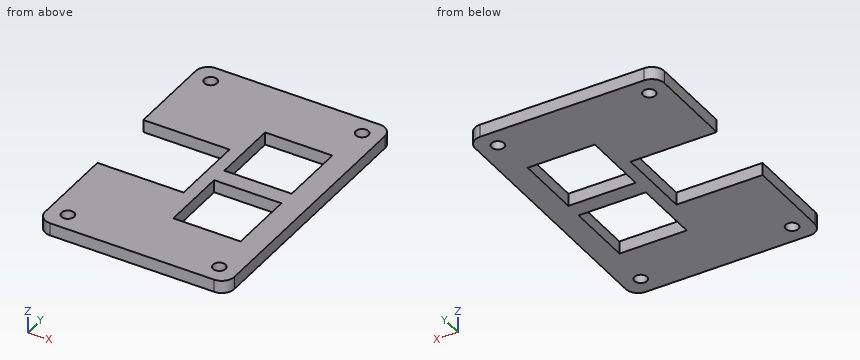
Autodesk Inventor part; units mm, degrees
ref_plane "YZ Plane" through (0, 0, 0) normal (1, 0, 0) x (0, 1, 0)
ref_plane "XZ Plane" through (0, 0, 0) normal (0, 1, 0) x (-1, 0, 0)
ref_plane "XY Plane" through (0, 0, 0) normal (0, 0, 1) x (1, 0, 0)
sketch "Эскиз1" plane through (0, 0, 0) normal (0, 0, 1) x (1, 0, 0)
  arc A0 (22.5, 29.5) -> (19.5, 32.5) centre (19.5, 29.5) ccw
  line L0 (22.5, -29.5) -> (22.5, 29.5)
  arc A1 (19.5, -32.5) -> (22.5, -29.5) centre (19.5, -29.5) ccw
  line L1 (-19.5, -32.5) -> (19.5, -32.5)
  line L2 (19.5, 32.5) -> (-19.5, 32.5)
  arc A2 (-19.5, 32.5) -> (-22.5, 29.5) centre (-19.5, 29.5) ccw
  line L3 (-22.5, 29.5) -> (-22.5, 9)
  line L4 (-22.5, -9) -> (-22.5, -29.5)
  arc A3 (-22.5, -29.5) -> (-19.5, -32.5) centre (-19.5, -29.5) ccw
  circle A4 centre (-18, -28) radius 1.5
  circle A5 centre (18, -28) radius 1.5
  circle A6 centre (18, 28) radius 1.5
  circle A7 centre (-18, 28) radius 1.5
  line L5 (-2, 9) -> (-20, 9)
  line L6 (-22.5, 9) -> (-20, 9)
  line L7 (-2, -9) -> (-2, 9)
  line L8 (-20, -9) -> (-2, -9)
  line L9 (-20, -9) -> (-22.5, -9)
  line L10 (1, -2) -> (1, -18)
  line L11 (1, -18) -> (17, -18)
  line L12 (17, -18) -> (17, -2)
  line L13 (17, -2) -> (1, -2)
  line L14 (1, 18) -> (1, 2)
  line L15 (1, 2) -> (17, 2)
  line L16 (17, 2) -> (17, 18)
  line L17 (17, 18) -> (1, 18)
  point P0 (0, 0)
extrude "Выдавливание1" add sketch "Эскиз1" along normal blind 3
properties part number "level2_up"
Can you work these out from the model? Positions are in its coordinate system, mm. Give positions to 0.01 mm unless a question says otherwise; leave off trailing zeros. Write each loop counter-clockwise with the first axis right and the second up, starting at its lowest first coordinate (ties: lowest second). Pieces come first, ordered by that corner, then holes. Notation, with made-up numbers: (-9.75, -31.75) -> (15.25, -31.75) arc R27 cw to (15.25, -3.75) -> close; hole circle Ø8 at (-27.75, -19). An arc over 180 degrees is marked (long way). Answer as a JSON object with one key per item and string values. Group by question number.
Item 1: I'm going to push flat-ended pins straight in: P1, Ø4, axis at x = 18, y = 28, coming from the +Z side; P2, Ø1.8, axis at x = 18, y = -28, coming from the +Z side (3 decimals); P3, Ø1.5, axis at y = 6, z = 1.5, coming from the -X side. Where does each tip first touch, or does it pass through?
Item 2: Suppose I cut it at A-A (y = 28). Please give me the cut outline in (x, z), plus the area to 3 significant figures.
Item 3: Suppose I cut it at D-D (y = 4). Please give me the cut outline in (x, z), plus the area to 3 significant figures.
Item 4: Please list where these lines run through material, in increasing order: line 1 (Y direction, x = 4, z = 1.4); line 2 (Y direction, x = -18, z = 2.3); line 3 (Y direction, x = 18, z = 2.25). Write a range as [from, to].
Item 5: Suppose I cut it at C-C (x = 18). Please give me the cut outline in (y, z).
Item 6: Suppose I cut it at B-B (x = -18). Please give me the cut outline in (y, z).
Findings:
{
 "1": {"P1": "stops at z = 3", "P2": "passes through", "P3": "stops at x = -2"},
 "2": {"outline": "(-22.5, 0) -> (-19.5, 0) -> (-19.5, 3) -> (-22.5, 3) -> close; (-16.5, 0) -> (16.5, 0) -> (16.5, 3) -> (-16.5, 3) -> close; (19.5, 0) -> (22.5, 0) -> (22.5, 3) -> (19.5, 3) -> close", "area": "117 mm²"},
 "3": {"outline": "(-2, 0) -> (1, 0) -> (1, 3) -> (-2, 3) -> close; (17, 0) -> (22.5, 0) -> (22.5, 3) -> (17, 3) -> close", "area": "25.5 mm²"},
 "4": {"line 1": "y = [-32.5, -18], [-2, 2], [18, 32.5]", "line 2": "y = [-32.5, -29.5], [-26.5, -9], [9, 26.5], [29.5, 32.5]", "line 3": "y = [-32.5, -29.5], [-26.5, 26.5], [29.5, 32.5]"},
 "5": {"outline": "(-32.5, 0) -> (-29.5, 0) -> (-29.5, 3) -> (-32.5, 3) -> close; (-26.5, 0) -> (26.5, 0) -> (26.5, 3) -> (-26.5, 3) -> close; (29.5, 0) -> (32.5, 0) -> (32.5, 3) -> (29.5, 3) -> close"},
 "6": {"outline": "(-32.5, 0) -> (-29.5, 0) -> (-29.5, 3) -> (-32.5, 3) -> close; (-26.5, 0) -> (-9, 0) -> (-9, 3) -> (-26.5, 3) -> close; (9, 0) -> (26.5, 0) -> (26.5, 3) -> (9, 3) -> close; (29.5, 0) -> (32.5, 0) -> (32.5, 3) -> (29.5, 3) -> close"}
}
